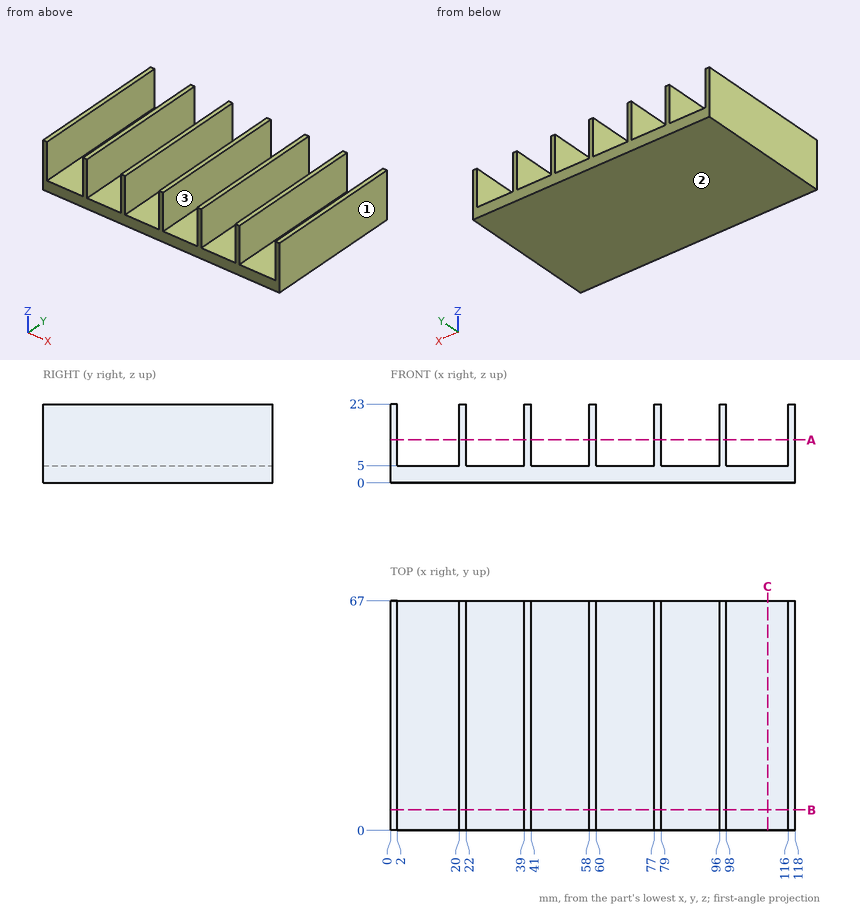
Check sheet for the drawn part. Datum: minimum x, y, z corner. Units: mm. Coordinates: 2 decimals unless noted, no trailing zeros. Write each loop counter-clockwise with the first axis right and the second up, starting at its lowest first coordinate (ties: lowest second). Pieces come first, ordered by that corner, then holes. Notation, with made-up numbers: M 33.25,20.5 L 92.25,20.5 A18 ccw 92.25,35.5 Z; hole C -17,56 d4. An arc over 180 degrees is marked long. Use a Markdown table: item, result.
Q1. Sectioned sample at A-A, the plane z = 12.5. Record the boundary of the cut face in (x, y).
Reply:
| item | result |
|---|---|
| outline | M 0,0 L 2,0 L 2,67 L 0,67 Z; M 20,0 L 22,0 L 22,67 L 20,67 Z; M 39,0 L 41,0 L 41,67 L 39,67 Z; M 58,0 L 60,0 L 60,67 L 58,67 Z; M 77,0 L 79,0 L 79,67 L 77,67 Z; M 96,0 L 98,0 L 98,67 L 96,67 Z; M 116,0 L 118,0 L 118,67 L 116,67 Z |
Q2. Go/stop test with a flat-tipped pin: P1, Ø2, axis at x = 70.5, y = 19, coming from the +Z side. Record where the tip stops, or that it passes through.
Reply:
| item | result |
|---|---|
| P1 | stops at z = 5 |
Q3. Thickness scan on line 1 (Z direction, x = 53, y = 62). Record the ranges inside material, lowest first.
Reply:
| item | result |
|---|---|
| line 1 | z = 0 to 5 |
Q4. Draft check along X on the marked faces 1, 2 and 3. Enter one of: +X half, -X half, draft (parallel to the pull), parting line (faces both ways), or undercut.
Reply:
| item | result |
|---|---|
| face 1 | +X half |
| face 2 | draft |
| face 3 | undercut |
Q5. Sectioned sample at C-C, the plane x = 110. Record the boundary of the cut face in (y, z), plus the area to 3 significant figures.
Reply:
| item | result |
|---|---|
| outline | M 0,0 L 67,0 L 67,5 L 0,5 Z |
| area | 335 mm² |
Q6. Sectioned sample at B-B, the plane y = 6. Record the boundary of the cut face in (x, z), plus the area to 3 significant figures.
Reply:
| item | result |
|---|---|
| outline | M 0,0 L 118,0 L 118,23 L 116,23 L 116,5 L 98,5 L 98,23 L 96,23 L 96,5 L 79,5 L 79,23 L 77,23 L 77,5 L 60,5 L 60,23 L 58,23 L 58,5 L 41,5 L 41,23 L 39,23 L 39,5 L 22,5 L 22,23 L 20,23 L 20,5 L 2,5 L 2,23 L 0,23 Z |
| area | 842 mm² |
